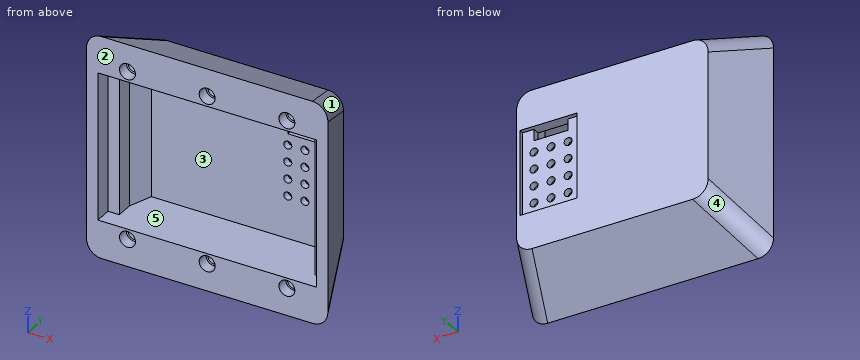
from build123d import *

# Parameters (mm, degrees)
TOP_ENCLOSURE_DEPTH                     = 65
TOP_EXTRA_DEPTH                         = 2.5
SKETCH3_W                               = 25
SKETCH3_H                               = 37.5
SOLAR_CELL_SLOT_DEPTH                   = 2
BOSS_EXTRUDE1_REACH                     = 91.819
BOSS_EXTRUDE2_REACH                     = 102.756
FILLET1_R                               = 7.5
CBORE_FOR_M5_HEX_HEAD_BOLT1_D           = 5.3
CBORE_FOR_M5_HEX_HEAD_BOLT1_DEPTH       = 10
CBORE_FOR_M5_HEX_HEAD_BOLT1_CBORE_D     = 7
CBORE_FOR_M5_HEX_HEAD_BOLT1_CBORE_DEPTH = 5
SKETCH10_R                              = 1.75
SKETCH10_W                              = 15
SKETCH10_H                              = 5
CUT_EXTRUDE1_DEPTH                      = 102.160736278


with BuildPart() as part:
    # Master_Geometry → Top_Enclosure (new body)
    with BuildSketch(Plane.XY):
        Polygon((-48, -3.5), (-53, -3.5), (-42.080892972, 26.5), (42.080892972, 26.5), (53, -3.5), (48, -3.5), (48, 4), (43, 4), (43, 11.5), (39.360297657, 21.5), (-39.360297657, 21.5), (-43, 11.5), (-43, 4), (-48, 4), align=None)
    extrude(amount=TOP_ENCLOSURE_DEPTH)

    # Sketch2 → Top_Extra (add)
    with BuildSketch(Plane.XY.offset(65)):
        Polygon((-42.080892972, 26.5), (42.080892972, 26.5), (53, -3.5), (-53, -3.5), align=None)
    top_extra = extrude(amount=TOP_EXTRA_DEPTH)

    # Mirror1: Top_Extra across plane
    add(top_extra.mirror(Plane(origin=(0, 0, 32.5), x_dir=(1, 0, 0), z_dir=(0, 0, -1))))

    # Sketch3 → Solar_Cell_Slot (cut)
    with BuildSketch(Plane(origin=(0, 26.5, 0), x_dir=(1, 0, 0), z_dir=(0, 1, 0))):
        with Locations((28.080892972, -32.5)):
            Rectangle(SKETCH3_W, SKETCH3_H)
    extrude(amount=-SOLAR_CELL_SLOT_DEPTH, mode=Mode.SUBTRACT)

    # Boss-Extrude1: up to this plane
    boss_extrude1_end = Plane(origin=(42.080892972, 26.5, 65), z_dir=(-0.9396926207859069, -0.3420201433256729, 0))
    # Sketch5 → Boss-Extrude1 (add, up to the surface)
    with BuildSketch(Plane(origin=(0, 0, 0), x_dir=(0, 0, -1), z_dir=(1, 0, 0)), mode=Mode.PRIVATE) as boss_extrude1_sk1:
        Polygon((-67.5, 26.5), (-67.5, -3.5), (-81.489229745, -3.5), align=None)
    boss_extrude1_tool1 = split(extrude(boss_extrude1_sk1.sketch, amount=BOSS_EXTRUDE1_REACH, mode=Mode.PRIVATE), bisect_by=boss_extrude1_end, keep=Keep.BOTH, mode=Mode.PRIVATE)
    boss_extrude1 = boss_extrude1_tool1.solids().sort_by_distance((0, 6.5, 72.163077))[0]
    add(boss_extrude1)

    # Boss-Extrude2: up to this face of the body (flat: up to its plane)
    boss_extrude2_end = Plane(part.part.faces().sort_by_distance((-47.540446486, 11.5, 32.5))[0])
    # Sketch6 → Boss-Extrude2 (add, up to the picked face)
    with BuildSketch(Plane.ZY, mode=Mode.PRIVATE) as boss_extrude2_sk1:
        Polygon((67.5, 26.5), (81.489229745, -3.5), (67.5, -3.5), align=None)
    boss_extrude2_tool1 = split(extrude(boss_extrude2_sk1.sketch, amount=BOSS_EXTRUDE2_REACH, mode=Mode.PRIVATE), bisect_by=boss_extrude2_end, keep=Keep.BOTH, mode=Mode.PRIVATE)
    boss_extrude2 = boss_extrude2_tool1.solids().sort_by(Axis((0, 6.5, 72.163077), (-1, 0, 0)))[0]
    add(boss_extrude2)

    # Mirror3: Boss-Extrude1, Boss-Extrude2 across plane
    add(boss_extrude1.mirror(Plane(origin=(0, 0, 32.5), x_dir=(1, 0, 0), z_dir=(0, 0, -1))))
    add(boss_extrude2.mirror(Plane(origin=(0, 0, 32.5), x_dir=(1, 0, 0), z_dir=(0, 0, -1))))

    # Fillet1
    fillet1_edges = [part.edges().sort_by_distance(p)[0] for p in [
        (47.540446486, 11.5, -9.494614872),
        (-47.540446486, 11.5, -9.494614872),
        (47.540446486, 11.5, 74.494614872),
        (-47.540446486, 11.5, 74.494614872),
    ]]
    fillet(fillet1_edges, radius=FILLET1_R)

    # CBORE for M5 Hex Head Bolt1
    with Locations(Plane(origin=(0, -3.5, 0), x_dir=(-1, 0, 0), z_dir=(0, -1, 0))):
        with Locations((35, -69.489229745), (0, -69.489229745), (-35, -69.489229745), (-35, 4.489229745), (0, 4.489229745), (35, 4.489229745)):
            CounterBoreHole(CBORE_FOR_M5_HEX_HEAD_BOLT1_D / 2, CBORE_FOR_M5_HEX_HEAD_BOLT1_CBORE_D / 2, CBORE_FOR_M5_HEX_HEAD_BOLT1_CBORE_DEPTH, depth=CBORE_FOR_M5_HEX_HEAD_BOLT1_DEPTH)

    # Sketch10 → Cut-Extrude1 (cut, through all)
    with BuildSketch(Plane(origin=(0, 24.5, 0), x_dir=(1, 0, 0), z_dir=(0, 1, 0))):
        with Locations(Location((20.580892972, -18.75, 0), (0, 0, 270))):
            Circle(SKETCH10_R)
        with Locations(Location((28.080892972, -18.75, 0), (0, 0, 270))):
            Circle(SKETCH10_R)
        with Locations(Location((35.580892972, -18.75, 0), (0, 0, 270))):
            Circle(SKETCH10_R)
        with Locations(Location((35.580892972, -26.25, 0), (0, 0, 270))):
            Circle(SKETCH10_R)
        with Locations(Location((28.080892972, -26.25, 0), (0, 0, 270))):
            Circle(SKETCH10_R)
        with Locations(Location((20.580892972, -26.25, 0), (0, 0, 270))):
            Circle(SKETCH10_R)
        with Locations(Location((35.580892972, -33.75, 0), (0, 0, 270))):
            Circle(SKETCH10_R)
        with Locations(Location((28.080892972, -33.75, 0), (0, 0, 270))):
            Circle(SKETCH10_R)
        with Locations(Location((20.580892972, -33.75, 0), (0, 0, 270))):
            Circle(SKETCH10_R)
        with Locations(Location((35.580892972, -41.25, 0), (0, 0, 270))):
            Circle(SKETCH10_R)
        with Locations(Location((28.080892972, -41.25, 0), (0, 0, 270))):
            Circle(SKETCH10_R)
        with Locations(Location((20.580892972, -41.25, 0), (0, 0, 270))):
            Circle(SKETCH10_R)
        with Locations((28.080892972, -48.75)):
            Rectangle(SKETCH10_W, SKETCH10_H)
    extrude(amount=-CUT_EXTRUDE1_DEPTH, mode=Mode.SUBTRACT)


solid = part.part
Could you check a few things on this model? Use its own coordinates, in mm. Face numbers are marked on the shaded views. A direction names the side the tool comes from. Give positions to 0.01 mm unless a question says otherwise; leave off trailing zeros. Order: outer loops, then holes, each group sorted by start corner. A loop starts at its lowest first (then second) coordinate and runs counter-clockwise, first axis right, second up.
1. We'd pull the mould along Z, two halves only. Please class the marked faces 1, 2 and 3: pulls with the +Z half, pulls with the -Z half, needs draft (parallel to the pull), parting line crosses it, or undercut.
2. Suppose I cut it at B-B (z = 53). List the corners of the cut face in (x, y) for me, plus the area to 3 significant figures.
3. Suppose I cut it at D-D (x = 0). List the corners of the cut face in (y, z) for me.
4. I need wall thicknesses on L1, parallel to X at y = 22, z = 33; L2, parallel to X at y = 23.25, z = 41.25; L3, parallel to Z at x = -35, y = 4.8. Which ranges of each line are inside material? Lowest first, please.
5. Suppose I cut it at C-C (x = -19). List the corners of the cut face in (y, z) for me, plus the area to 3 significant figures.
6. Will these pins go through, and if not, where does the flat tip stop? P1, Ø1, axis at x = 6.5, z = 62, coming from the -Y side; P2, Ø6, axis at y = 7.5, z = 26.5, coming from the -X side; P3, Ø5, axis at x = -33.5, y = 11, coming from the +Z side; P4, Ø9, axis at x = 35, z = -4.49, coming from the -Y side.
7. Suppose I cut it at A-A (z = 33.75). Give the number of separate pieces and of enclosed holes in the cut face, plus the area to 3 significant figures.
8. For the marked faces 4 and 5, which set-ups out of +Z, -Z, +X, -X, +Y, -Y let a thin tool reach every point of the face, with its end or its side?
Solved:
1. face 1: pulls with the +Z half
1. face 2: needs draft
1. face 3: undercut
2. outline: (-53, -3.5) - (-48, -3.5) - (-48, 4) - (-43, 4) - (-43, 11.5) - (-39.36, 21.5) - (39.36, 21.5) - (43, 11.5) - (43, 4) - (48, 4) - (48, -3.5) - (53, -3.5) - (42.08, 26.5) - (-42.08, 26.5) - close
2. area: 664 mm2
3. outline: (-3.5, -16.49) - (26.5, -2.5) - (26.5, 67.5) - (-3.5, 81.49) - (-3.5, 72.99) - (1.5, 72.99) - (1.5, 72.14) - (6.5, 72.14) - (6.5, 66.84) - (1.5, 66.84) - (1.5, 65.99) - (-3.5, 65.99) - (-3.5, 65) - (21.5, 65) - (21.5, 0) - (-3.5, 0) - (-3.5, -0.99) - (1.5, -0.99) - (1.5, -1.84) - (6.5, -1.84) - (6.5, -7.14) - (1.5, -7.14) - (1.5, -7.99) - (-3.5, -7.99) - close
4. L1: x = -43.72 to 19, 22.16 to 26.5, 29.66 to 34, 37.16 to 43.72
4. L2: x = -43.26 to 18.83, 22.33 to 26.33, 29.83 to 33.83, 37.33 to 43.26
4. L3: z = -12.62 to -7.14, -1.84 to 0, 65 to 66.84, 72.14 to 77.62
5. outline: (-3.5, -16.49) - (26.5, -2.5) - (26.5, 67.5) - (-3.5, 81.49) - (-3.5, 65) - (21.5, 65) - (21.5, 0) - (-3.5, 0) - close
5. area: 895 mm2
6. P1: stops at y = 21.5
6. P2: stops at x = -50.09
6. P3: stops at z = 75.89
6. P4: stops at y = -3.5
7. separate pieces: 4
7. enclosed holes: 0
7. area: 582 mm2
8. face 4: -Z, -X, +Y
8. face 5: -Y
